from build123d import *

# Parameters (mm, degrees)
SKETCH3_R           = 317.5
BOSS_EXTRUDE2_DEPTH = 100
FILLET5_R           = 20
SKETCH4_R           = 63.5
SKETCH4_R_2         = 50.8
BOSS_EXTRUDE3_DEPTH = 10


with BuildPart() as part:
    # Sketch3 → Boss-Extrude2 (new body)
    with BuildSketch(Plane(origin=(0, 0, 0), x_dir=(1, 0, 0), z_dir=(0, 1, 0))):
        with Locations(Location((0, 0, 0), (0, 0, 270))):
            Circle(SKETCH3_R)
    extrude(amount=BOSS_EXTRUDE2_DEPTH)

    # Fillet5
    fillet5_edges = [part.edges().sort_by_distance(p)[0] for p in [
        (0, 0, -317.5),
        (0, 100, -317.5),
    ]]
    fillet(fillet5_edges, radius=FILLET5_R)

    # Sketch4 → Boss-Extrude3 (add)
    with BuildSketch(Plane(origin=(0, 0, 0), x_dir=(1, 0, 0), z_dir=(0, 1, 0))):
        with Locations(Location((0, 0, 0), (0, 0, 270))):
            Circle(SKETCH4_R)
        with Locations(Location((0, 0, 0), (0, 0, 270))):
            Circle(SKETCH4_R_2, mode=Mode.SUBTRACT)
    extrude(amount=-BOSS_EXTRUDE3_DEPTH)


solid = part.part
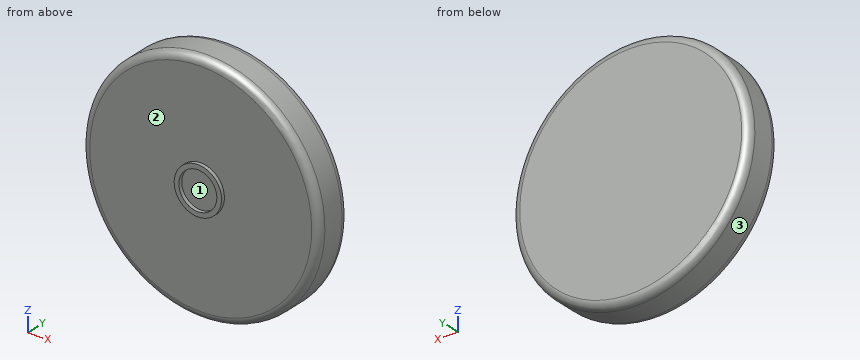
Geometry check sheet. Reference: the model listing, model coordinates, mm. Face numbers are marked on the shaded views. Round coordinates to 2 decimals unless told otherwise and drop trailing zeros. Order: outer loops, then holes, each group sorted by start corner. A loop starts at its lowest first (then second) coordinate and runs counter-clockwise, first axis right, second up. Notation, with made-up numbers: (8, -34) -> (17, -34) arc R30 ccw to (17, -5) -> close; hole circle Ø2 at (56.5, 23.25). An arc over 180 degrees is marked (long way). Use one line per item in the form item = value.
1. Go/stop test with flat-tipped pins: pin 1 (10 mm diameter, centred on y = 1.5, z = -250, fed in from +X); pin 2 (2 mm diameter, centred on x = 125, y = 73.5, fed in from -Z); pin 3 (10 mm diameter, centred on y = 4, z = 37, fed in from +X). Record where each tip stops, or that it passes through.
Working result:
pin_1 = 189.43
pin_2 = -292.28
pin_3 = 312.07
2. Cross-section at A-A, the plane z = 0. Enter the section's corners in (x, y).
Working result:
outline = (-317.5, 20) arc R20 ccw to (-297.5, 0) -> (-63.5, 0) -> (-63.5, -10) -> (-50.8, -10) -> (-50.8, 0) -> (50.8, 0) -> (50.8, -10) -> (63.5, -10) -> (63.5, 0) -> (297.5, 0) arc R20 ccw to (317.5, 20) -> (317.5, 80) arc R20 ccw to (297.5, 100) -> (-297.5, 100) arc R20 ccw to (-317.5, 80) -> close
3. Cross-section at B-B, the plane x = 0. Enter the section's corners in (y, z).
Working result:
outline = (-10, -63.5) -> (0, -63.5) -> (0, -297.5) arc R20 ccw to (20, -317.5) -> (80, -317.5) arc R20 ccw to (100, -297.5) -> (100, 297.5) arc R20 ccw to (80, 317.5) -> (20, 317.5) arc R20 ccw to (0, 297.5) -> (0, 63.5) -> (-10, 63.5) -> (-10, 50.8) -> (0, 50.8) -> (0, -50.8) -> (-10, -50.8) -> close
4. Cross-section at C-C, the plane y = 44. Enter the section's corners in (x, z), plus the area to 3 significant figures.
Working result:
outline = circle Ø635 at (0, 0)
area = 317,000 mm^2
5. Mould release check, pull along Z, two halves, no side actions. Record for the marked faces 1, 2 and 3: pulls with the +Z half, pulls with the -Z half, needs draft (parallel to the pull), parting line crosses it, or undercut.
Working result:
face_1 = undercut
face_2 = needs draft
face_3 = parting line crosses it
6. Cross-section at D-D, the plane y = 88.5. Enter the section's corners in (x, z).
Working result:
outline = circle Ø631.21 at (0, 0)
7. Scan lines: line 1 along X through (y, z) = (-2, 0); line 2 along Y through (x, z) = (86, 86); line 3 along X through (y, z) = (26, 0). Record each from-to range of solid material in increasing order. Write a range as from..to.
Working result:
line_1 = -63.5..-50.8, 50.8..63.5
line_2 = 0..100
line_3 = -317.5..317.5
